Verification items for the finished model (mm, model axes). Round coordinates to 2 decimals unless told otherwise and drop trailing zeros. Write each loop counter-clockwise with the first axis right and the second up, starting at its lowest first coordinate (ties: lowest second). Pieces come first, ordered by that corner, then holes. Notation, with made-up numbers: M 68,-36.5 L 86,-36.5 A20 cw 86,-10.5 Z; hole C 56.5,-9.5 d6. An arc over 180 degrees is marked long. One line per question, with ' | ' between items. Start each with the question number.
Q1. Cross-section at C-C (x = 0). Record the boundary of the cut face in (y, z), then the cut area to 3 significant figures.
Q2. Release check for a two-part mould opening along X. For faces 1 (the face through (-2.257, 3.405, -2.934)), 2 (the face through (-2.08, 3.69, -2.93)) record: released by +X, released by -X, zero draft, split by the parting line, or undercut.
Q3. Gauge pin test, flat end, axial feed: pin 1 (2 mm diameter, centred on x = 3, z = -2.5, fed in from +Y). Record the tip position at first contact, or that the pin passes through.
Q4. Cross-section at A-A (z = -3.45). Record the boundary of the cut face in (x, y) (3 decimals).
Q5. Thickness scan on line 1 along Y through (x, z) = (1.75, -0.7); line 2 along Y through (x, z) = (-2.25, -2.5); line 3 along X through (y, z) = (2.2, -2.3). Record the ranges inside material, lowest first. Write a range as from..to.
Q6. Cross-section at B-B (y = 3.7). Record the boundary of the cut face in (x, z), then the cut area to 3 significant figures.
from build123d import *

# Parameters (mm, degrees)
BASE_FLANGE1_DEPTH      = 2.4
BASE_FLANGE1_DEPTH_BACK = 2.4


# Sheet-metal steps are written as plain solids
with BuildPart() as part:
    # Sketch2 → Base-Flange1 (new, two sides: drawn at the far end of the back side and taken through both)
    with BuildSketch(Plane.XY.offset(-2.9).offset(-BASE_FLANGE1_DEPTH_BACK)):
        with BuildLine():
            Line((-7.675, 3.9), (3.315435248, 2.895852113))
            ThreePointArc((3.315435248, 2.895852113), (3.963023803, 2.574171105), (4.224448606, 1.9))
            Line((4.224448606, 1.9), (4.524448606, 1.9))
            ThreePointArc((4.524448606, 1.9), (4.184596362, 2.776422437), (3.342731241, 3.194607747))
            Line((3.342731241, 3.194607747), (-7.647704007, 4.198755634))
            Line((-7.647704007, 4.198755634), (-7.675, 3.9))
        make_face()
    extrude(amount=BASE_FLANGE1_DEPTH + BASE_FLANGE1_DEPTH_BACK)


solid = part.part
Determined:
1) outline: M 3.2,-5.3 L 3.5,-5.3 L 3.5,-0.5 L 3.2,-0.5 Z | area: 1.45 mm²
2) face 1: released by -X | face 2: released by +X
3) pin 1: stops at y = 3.32
4) outline: M -7.675,3.9 L 3.315,2.896 A1 cw 4.224,1.9 L 4.524,1.9 A1.3 ccw 3.343,3.195 L -7.648,4.199 Z
5) line 1: y = 3.04..3.34 | line 2: y = 3.4..3.71 | line 3: x = 4.18..4.49
6) outline: M -5.49,-5.3 L -2.19,-5.3 L -2.19,-0.5 L -5.49,-0.5 Z | area: 15.8 mm²
